from build123d import *

# Parameters (mm, degrees)
SKETCH_1_R               = 18
EXTRUDE_1_DEPTH          = 40
SKETCH_2_R               = 11
EXTRUDE_2_DEPTH          = 2
SKETCH_3_R               = 4
EXTRUDE_3_DEPTH          = 20
SKETCH_4_R               = 1.5
CUT_EXTRUDE_1_DEPTH      = 5
PATTERN_CIRCULAR_1_COUNT = 4
CUT_EXTRUDE_START        = -15
CUT_EXTRUDE_2_DEPTH      = 15
SKETCH_6_R               = 18.5
EXTRUDE_4_DEPTH          = 57


with BuildPart() as part:
    # 草图1 → 凸台-拉伸1 (new body)
    with BuildSketch(Plane(origin=(0, 0, 0), x_dir=(0, 0, -1), z_dir=(1, 0, 0))):
        Circle(SKETCH_1_R)
    extrude(amount=EXTRUDE_1_DEPTH)

    # 草图2 → 凸台-拉伸2 (add)
    with BuildSketch(Plane.ZY):
        Circle(SKETCH_2_R)
    extrude(amount=EXTRUDE_2_DEPTH)

    # 草图3 → 凸台-拉伸3 (add)
    with BuildSketch(Plane.ZY.offset(2)):
        Circle(SKETCH_3_R)
    extrude(amount=EXTRUDE_3_DEPTH)

    # 草图4 → 切除-拉伸1 (cut)
    with BuildSketch(Plane.ZY):
        with Locations((-14, 0)):
            Circle(SKETCH_4_R)
    cut_extrude_1 = extrude(amount=-CUT_EXTRUDE_1_DEPTH, mode=Mode.SUBTRACT)

    # 阵列(圆周)1: 切除-拉伸1 ×4 about axis
    pattern_circular_1_axis = Axis((0, 0, 0), (1, 0, 0))
    for i in range(1, PATTERN_CIRCULAR_1_COUNT):
        add(cut_extrude_1.rotate(pattern_circular_1_axis, i * 360 / PATTERN_CIRCULAR_1_COUNT), mode=Mode.SUBTRACT)

    # 草图5 → 切除-拉伸2 (cut)
    with BuildSketch(Plane.ZY.offset(22).offset(CUT_EXTRUDE_START)):
        with BuildLine():
            Line((-3.773069257, -1.328137186), (1.382044823, -3.753658496))
            ThreePointArc((1.382044823, -3.753658496), (-1.702949755, -3.619386983), (-3.773069257, -1.328137186))
        make_face()
    extrude(amount=CUT_EXTRUDE_2_DEPTH, mode=Mode.SUBTRACT)

    # 草图6 → 凸台-拉伸4 (add)
    with BuildSketch(Plane(origin=(40, 0, 0), x_dir=(0, 0, -1), z_dir=(1, 0, 0))):
        with Locations(Location((0, 0, 0), (0, 0, 180))):
            Circle(SKETCH_6_R)
    extrude(amount=EXTRUDE_4_DEPTH)


solid = part.part
Geometry check sheet. Reference: the model listing, model coordinates, mm. A direction names the side the tool comes from. Give positions to 0.01 mm unless a question says otherwise; leave off trailing zeros. Order: outer loops, then holes, each group sorted by start corner. A loop starts at its lowest first (then second) coordinate and runs counter-clockwise, first axis right, second up. Notation, with made-up numbers: M -27.75,-28.5 L -2.75,-28.5 A23 ccw -2.75,-3.5 Z; hole C 81,62.25 d2. An arc over 180 degrees is marked long. Use a Markdown table: item, result.
Item 1: Section check B-B (z = -7). Record the cut outline in (x, y).
Answers follow:
| item | result |
|---|---|
| outline | M -2,-8.49 L 0,-8.49 L 0,-16.58 L 40,-16.58 L 40,-17.12 L 97,-17.12 L 97,17.12 L 40,17.12 L 40,16.58 L 0,16.58 L 0,8.49 L -2,8.49 Z |
Item 2: Section check C-C (x = 60.5). Record the cut outline in (y, z).
Answers follow:
| item | result |
|---|---|
| outline | C 0,0 d37 |
Item 3: Tool access check on faces 4 (the flat face through (97, 0, 0)), 5 (the flat face through (5, 14, 0)), 6 (the flat face through (-7, -3, -1)). Record the directions out of +Z, -Z, +X, -X, +Y, -Y that give a thin tool (end or side, any length) a straight path to the whole face; none if there is none.
Answers follow:
| item | result |
|---|---|
| face 4 | +Z, -Z, +X, +Y, -Y |
| face 5 | -X |
| face 6 | -Z, -X, -Y |
Item 4: Draft check along Y on faces 1 (the cylindrical face through (2.46, -15.5, -0.07)), 2 (the flat face through (0, -8, 8)), 3 (the cylindrical face through (19.72, 17.847, 2.343)). Enter one of: +Y half, -Y half, draft (parallel to the pull), parting line (faces both ways), or undercut.
Answers follow:
| item | result |
|---|---|
| face 1 | undercut |
| face 2 | draft |
| face 3 | parting line |
Item 5: Depth check by flat-ended pin: P1, Ø8, axis at x = -2.5, z = -13, coming from the -Y side; P2, Ø1.5, axis at y = -0.5, z = -13.5, coming from the -X side; P3, Ø3.5, axis at y = 0, z = 13.5, coming from the -X side. Enter the tip coordinate at first touch or a pass-through.
Answers follow:
| item | result |
|---|---|
| P1 | stops at y = -15.05 |
| P2 | stops at x = 5 |
| P3 | stops at x = 0 |
Item 6: Section check D-D (y = 6). Record the cut outline in (x, z).
Answers follow:
| item | result |
|---|---|
| outline | M -2,-9.22 L 0,-9.22 L 0,-16.97 L 40,-16.97 L 40,-17.5 L 97,-17.5 L 97,17.5 L 40,17.5 L 40,16.97 L 0,16.97 L 0,9.22 L -2,9.22 Z |
Item 7: Material ranges on line 1 along X through (y, z) = (4.5, 12); line 2 along X through (y, z) = (6.5, -3); line 3 along Z through (x, y) = (3, 14), recorded low to high.
Answers follow:
| item | result |
|---|---|
| line 1 | x = 0 to 97 |
| line 2 | x = -2 to 97 |
| line 3 | z = -11.31 to -1.5, 1.5 to 11.31 |
Item 8: Section check A-A (y = 0). Record the cut outline in (x, z).
Answers follow:
| item | result |
|---|---|
| outline | M -22,-4 L -2,-4 L -2,-11 L 0,-11 L 0,-12.5 L 5,-12.5 L 5,-15.5 L 0,-15.5 L 0,-18 L 40,-18 L 40,-18.5 L 97,-18.5 L 97,18.5 L 40,18.5 L 40,18 L 0,18 L 0,15.5 L 5,15.5 L 5,12.5 L 0,12.5 L 0,11 L -2,11 L -2,4 L -22,4 Z |
